Can you work these out from the drawing? Everything is in mm from the part's minimum corner. Give positions to 0.01 mm unless a question says otherwise; leave off trailing zeros. Loops run counter-clockwise (first coordinate to the right, second up) from the corner with the lowest first, then second, coordinate; pieces in that order, holes last. Notation, with made-up numbers: M 33.5,88 L 73.5,88 A21 cw 73.5,126 Z; hole C 80.5,77.5 d3. An arc over 180 degrees is marked long. Use CSV: the item, a comma, the result in double quotes.
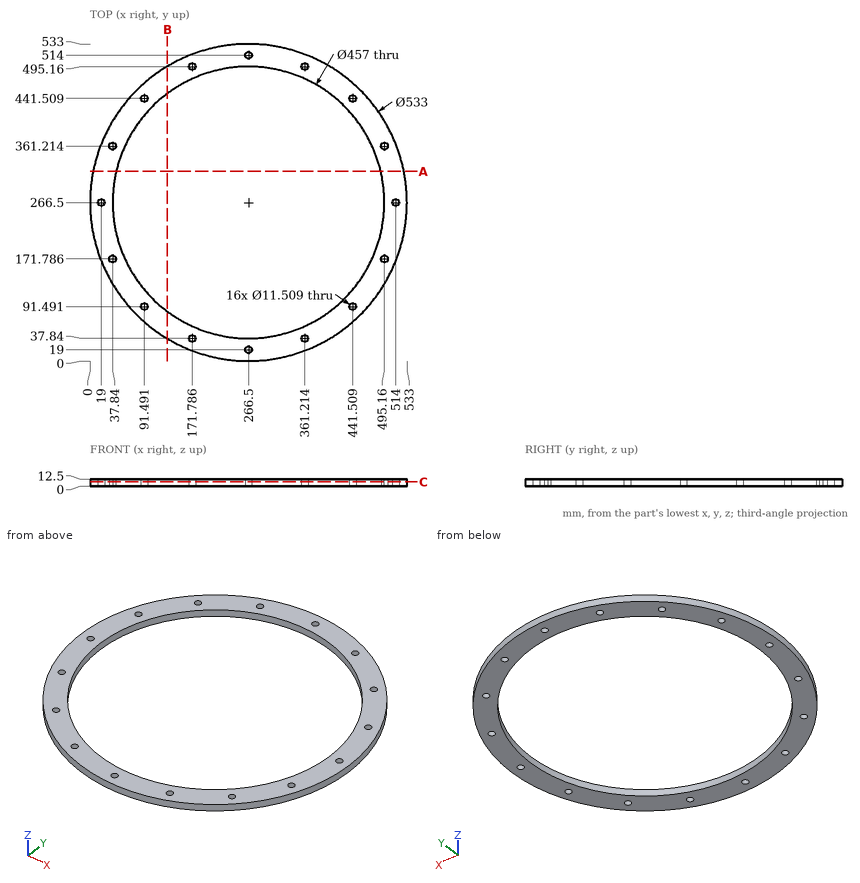
Q1. Please list where these lines run through material, in increasing order: L1, parallel to X at y = 364, z = 10.75 (1 decimal); L2, parallel to X at y = 36.5, z = 3.75; L3, parallel to X at y = 173.5, z = 2.5. Write a range as from..to.
Model answer:
L1,"18.5..32.8, 42.9..59.8, 473.2..490.1, 500.2..514.5"
L2,"131.88..166.19, 177.38..355.62, 366.81..401.12"
L3,"16.75..32.35, 43.33..57.78, 475.22..489.67, 500.65..516.25"
Q2. I'm going to push flat-ended pins straight in: P1, Ø2, axis at x = 361.5, z = 6, coming from the +Y side; P2, Ø2, axis at y = 112, z = 2.5, coming from the -X side; P3, Ø3, axis at y = 314, z = 4, coming from the -X side. Where does each tip first touch, or does it pass through?
Model answer:
P1,"y = 515.87"
P2,"x = 48.65"
P3,"x = 4"
Q3. I want a section at A-A, the plane y = 319. Please give me the cut outline in (x, z), then the cut area to 3 significant figures.
Model answer:
outline,"M 5.22,0 L 44.11,0 L 44.11,12.5 L 5.22,12.5 Z; M 488.89,0 L 527.78,0 L 527.78,12.5 L 488.89,12.5 Z"
area,"972 mm2"
Q4. I want a section at B-B, the plane x = 130. Please give me the cut outline in (y, z), then the cut area to 3 significant figures.
Model answer:
outline,"M 37.61,0 L 83.25,0 L 83.25,12.5 L 37.61,12.5 Z; M 449.75,0 L 495.39,0 L 495.39,12.5 L 449.75,12.5 Z"
area,"1,140 mm2"
Q5. I want a section at C-C, the plane z = 7.5. State how many separate pieces and enclosed holes the cut face has, then the cut area to 3 significant figures.
Model answer:
separate pieces,"1"
enclosed holes,"17"
area,"57,400 mm2"
